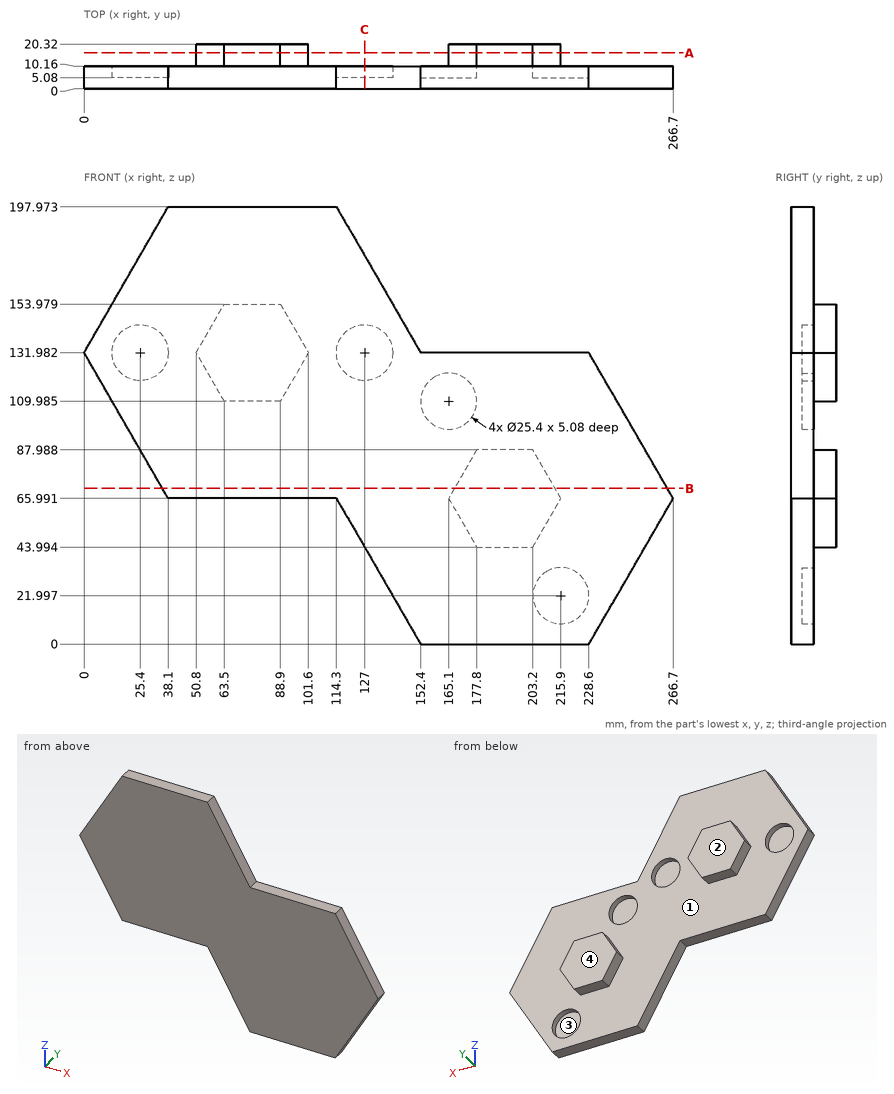
Input: dimensioned drawing with shaded views. Units: mm. Origin: part minimum x, y, z. A direction names the side the tool comes from. Give positions to 0.01 mm unless a question says otherwise; leave off trailing zeros. Order: outer loops, then holes, each group sorted by start corner. A loop starts at its lowest first (then second) coordinate and runs counter-clockwise, first axis right, second up.
(1) Section query C-C (x = 127). Return the cut outline in (y, z).
(2) Access query for the marked faces 1 and 2. Directions: +Z, -Z, +X, -X, +Y, -Y. A direction counts if a zero-diameter tool reaches every point of the face in a straight line with its end or side. Return the directions, or none.
(3) Pull-direction query (X, two-part tool) for the marked faces 3 and 4; classes: +X half, -X half, draft (parallel to the pull), parting line (faces both ways), or undercut.
(4) Material intervals for line 1 along Z through (x, y) = (165.1, 6.4) (1 decimal); line 2 along Z through (x, y) = (215.9, 8.65); line 3 along X through (y, z) = (8, 132.5), sorted ascending.
(5) Section query A-A (y = 16.25). Return the cut outline in (x, z) (1 decimal).
(6) Contact query for flat-ended pins moving along their axis: P1, Ø11, axis at x = 191.5, y = 16.5, coming from the -Z side; P2, Ø7.5, axis at x = 212, z = 28.5, coming from the +Y side; P3, Ø4, axis at y = 10.5, z = 60, coming from the +X side; P4, Ø1.5, axis at x = 51.5, z = 148.5, coming from the -Y side. Output: stop coordinate, or through.
(7) Section query B-B (z = 70.5). Return the cut outline in (x, y), plus the area to 3 significant figures.
Outcome:
1. outline: (0, 43.99) - (10.16, 43.99) - (10.16, 119.28) - (5.08, 119.28) - (5.08, 144.68) - (10.16, 144.68) - (10.16, 175.98) - (0, 175.98) - close
2. face 1: +Y
2. face 2: +Z, -Z, +X, -X, +Y
3. face 3: undercut
3. face 4: draft
4. line 1: z = 0 to 97.3, 122.7 to 132
4. line 2: z = 0 to 9.3, 34.7 to 131.98
4. line 3: x = 0.3 to 12.71, 38.09 to 114.31, 139.69 to 152.1
5. outline: (50.8, 132) - (63.5, 110) - (88.9, 110) - (101.6, 132) - (88.9, 154) - (63.5, 154) - close; (165.1, 66) - (177.8, 44) - (203.2, 44) - (215.9, 66) - (203.2, 88) - (177.8, 88) - close
6. P1: stops at z = 43.99
6. P2: stops at y = 5.08
6. P3: stops at x = 264.38
6. P4: stops at y = 0
7. outline: (35.5, 0) - (264.1, 0) - (264.1, 10.16) - (213.3, 10.16) - (213.3, 20.32) - (167.7, 20.32) - (167.7, 10.16) - (35.5, 10.16) - close
7. area: 2,790 mm2
